The model under review builds one solid part; all positions refer to its coordinate system, in mm. A direction names the side the tool comes from. Coordinates: 2 decimals unless noted, no trailing zeros. Write each loop counter-clockwise with the first axis right and the second up, starting at its lowest first coordinate (ties: lowest second). Pieces come first, ordered by that corner, then holes. Notation, with made-up numbers: (-18.75, 22) -> (24.25, 22) arc R16 ccw to (24.25, 42) -> close; hole circle Ø1 at (25.25, 22). An arc over 180 degrees is marked (long way). Put each result on its own line as item: value. Start each with the question number.
from build123d import *

# Parameters (mm, degrees)
PAD_DEPTH       = 10
SKETCH001_W     = 26
SKETCH001_H     = 16
POCKET_DEPTH    = 8
SKETCH002_W     = 10
SKETCH002_H     = 2
POCKET001_DEPTH = 1.5


with BuildPart() as part:
    # Sketch → Pad (new body)
    with BuildSketch(Plane.XY):
        Polygon((15, 10), (15, -10), (5, -10), (5, -8.5), (-5, -8.5), (-5, -10), (-15, -10), (-15, 10), (-5, 10), (-5, 8.5), (5, 8.5), (5, 10), align=None)
    extrude(amount=PAD_DEPTH)

    # Sketch001 (on Face13 of Pad) → Pocket (cut)
    with BuildSketch(Plane(origin=(0, 0, 0), x_dir=(1, 0, 0), z_dir=(0, 0, -1))):
        Rectangle(SKETCH001_W, SKETCH001_H)
    extrude(amount=-POCKET_DEPTH, mode=Mode.SUBTRACT)

    # Sketch002 (on Face5 of Pocket) → Pocket001 (cut)
    with BuildSketch(Plane.XY.offset(10)):
        with Locations((0, 7.5)):
            Rectangle(SKETCH002_W, SKETCH002_H)
        with Locations((0, -7.5)):
            Rectangle(SKETCH002_W, SKETCH002_H)
    extrude(amount=-POCKET001_DEPTH, mode=Mode.SUBTRACT)


solid = part.part
1. Insertion check: P1, Ø6, axis at x = -4.5, z = 4.5, coming from the -Y side; P2, Ø0.6, axis at x = 1.5, y = -7.5, coming from the +Z side; P3, Ø1.2, axis at x = -1.5, z = 9, coming from the +Y side; P4, Ø1.2, axis at x = -1.5, z = 9, coming from the -Y side. Each pin has a flat end and moves straight along its axis. Give the tip position at first contact, or say it passes through.
2. Tool access review of faces 1 (the flat face through (0, -8, 4)), 2 (the flat face through (0, -8.5, 4)), 3 (the flat face through (-5, 9, 5)), 4 (the flat face through (0, -6.5, 9)), 5 (the flat face through (0, 0, 10)): name each direction out of +Z, -Z, +X, -X, +Y, -Y from which nothing blocks a thin tool from reaching the whole face with its end or side.
3. The part is to be moulded in two halves that separate along X. For faces 6 (the flat face through (10, -10, 5)), 7 (the flat face through (-15, 0, 5)), 8 (the flat face through (15, 0, 5)), 9 (the flat face through (0, -7, 8.5)), say which applies: released by +X, released by -X, zero draft, split by the parting line, or undercut.
4. Consider section B-B on x = -10.5. State the section outline as (y, z) points, then the cut area to 3 significant figures.
5. Wall thickness on line 1 (X direction, y = -2.75, z = 5.5); line 2 (Y direction, x = 2, z = 0.75); line 3 (Y direction, x = 8.5, z = 1): over which ranges is each line inside the solid? List them lowest first. Write a range as from..to.
6. Consider section A-A on z = 6.25. State the section outline as (x, y) points.
7. Consider section D-D on z = 9.25. State the section outline as (x, y) points, then the cut area to 3 significant figures.
8. Consider section C-C on y = -1.5. State the section outline as (x, z) points, then the cut area to 3 significant figures.
Output values:
1. P1: stops at y = -10
1. P2: stops at z = 8.5
1. P3: stops at y = 8.5
1. P4: stops at y = -8.5
2. face 1: -Z
2. face 2: +Z, -Z, -Y
2. face 3: +Z, +Y
2. face 4: +Z, -Y
2. face 5: +Z, +X, -X, +Y, -Y
3. face 6: zero draft
3. face 7: released by -X
3. face 8: released by +X
3. face 9: undercut
4. outline: (-10, 0) -> (-8, 0) -> (-8, 8) -> (8, 8) -> (8, 0) -> (10, 0) -> (10, 10) -> (-10, 10) -> close
4. area: 72.0 mm^2
5. line 1: x = -15..-13, 13..15
5. line 2: y = -8.5..-8, 8..8.5
5. line 3: y = -10..-8, 8..10
6. outline: (-15, -10) -> (-5, -10) -> (-5, -8.5) -> (5, -8.5) -> (5, -10) -> (15, -10) -> (15, 10) -> (5, 10) -> (5, 8.5) -> (-5, 8.5) -> (-5, 10) -> (-15, 10) -> close; hole (-13, -8) -> (13, -8) -> (13, 8) -> (-13, 8) -> close
7. outline: (-15, -10) -> (-5, -10) -> (-5, -6.5) -> (5, -6.5) -> (5, -10) -> (15, -10) -> (15, 10) -> (5, 10) -> (5, 6.5) -> (-5, 6.5) -> (-5, 10) -> (-15, 10) -> close
7. area: 530 mm^2
8. outline: (-15, 0) -> (-13, 0) -> (-13, 8) -> (13, 8) -> (13, 0) -> (15, 0) -> (15, 10) -> (-15, 10) -> close
8. area: 92.0 mm^2
